The listing builds one solid part. Answer for the finished solid, in the listing's coordinates (mm). A direction names the side the tool comes from. Give positions to 0.01 mm unless a question says otherwise; leave off trailing zeros. Write each loop counter-clockwise with the first axis right and the second up, starting at its lowest first coordinate (ties: lowest second). Pieces come first, ordered by that corner, then holes. Notation, with made-up numbers: (-3, 38.25) -> (39, 38.25) arc R16 cw to (39, 50.25) -> close; hole circle Ø5 at (62.25, 64). An arc over 180 degrees is marked (long way). Write each question's results on one line, items separated by ' | '. Start each with the question number.
from build123d import *

# Parameters (mm, degrees)
F0_R      = 3.15
F1_DEPTH  = 13
F3_DEPTH  = 5.25
F5_DEPTH  = 5.5
F6_R      = 5.05
F7_DEPTH  = 5.5
F13_ANGLE = 45
F14_DEPTH = 15.67431457


# Not quite as in the source:
# - ends of sketch curves that miss each other by under 0.0002 mm in the source are joined


with BuildPart() as f1:
    # F0 (on Right) → F1 (new body, symmetric)
    with BuildSketch(Plane.YZ):
        with BuildLine():
            ThreePointArc((0.206929, -7.128644), (-5.293071, -1.628644), (0.206929, 3.871356))
            Line((0.206929, 3.871356), (17.0618508568, 3.871356))
            ThreePointArc((17.0618508568, 3.871356), (18.7952856408, 4.1814515394), (20.3137082671, 5.0732744602))
            Line((20.3137082671, 5.0732744602), (32.8624566897, 15.8173146076))
            ThreePointArc((32.8624566897, 15.8173146076), (34.1525860171, 17.5248563908), (34.6105992794, 19.6153961475))
            Line((34.6105992794, 19.6153961475), (34.6105992794, 22.815095))
            Line((34.6105992794, 22.815095), (30.788173, 22.815095))
            ThreePointArc((30.788173, 22.815095), (25.288173, 28.315095), (30.788173, 33.815095))
            Line((30.788173, 33.815095), (18.7829781294, 33.815095))
            ThreePointArc((18.7829781294, 33.815095), (17.4423484261, 33.6320143473), (16.1998960673, 33.0961797995))
            Line((16.1998960673, 33.0961797995), (-17.01485, 13.055368))
            ThreePointArc((-17.01485, 13.055368), (-20.6995911511, -1.839295663), (-32.9318010984, -11.1021976908))
            ThreePointArc((-32.9318010984, -11.1021976908), (-39.5666476125, -27.8428278397), (-21.8415422013, -31.0193857649))
            Line((-21.8415422013, -31.0193857649), (6.062198, -7.128644))
            Line((6.062198, -7.128644), (0.206929, -7.128644))
        make_face()
        with Locations((-29.405486, -22.184905)):
            Circle(F0_R, mode=Mode.SUBTRACT)
    extrude(amount=F1_DEPTH, both=True)

    # F2 (on Right) → F3 (cut, symmetric)
    with BuildSketch(Plane.YZ):
        with BuildLine():
            ThreePointArc((-21.905486, -3.502726), (-26.8533127567, -8.1227182817), (-32.9318011292, -11.1021976663))
            ThreePointArc((-32.9318011292, -11.1021976663), (-39.5869945241, -27.806130876), (-21.905486, -31.0737348541))
            Line((-21.905486, -31.0737348541), (-21.905486, -3.502726))
        make_face()
    extrude(amount=F3_DEPTH, both=True, mode=Mode.SUBTRACT)

    # F4 (on face) → F5 (cut)
    with BuildSketch(Plane.YZ.offset(13)):
        Polygon((-26.8555401867, -27.4290550439), (-23.5889459341, -22.5986621693), (-26.1388917474, -17.3545121255), (-31.9554318133, -16.9407549561), (-35.2220260659, -21.7711478307), (-32.6720802526, -27.0152978745), align=None)
    extrude(amount=-F5_DEPTH, mode=Mode.SUBTRACT)

    # F6 (on face) → F7 (cut)
    with BuildSketch(Plane(origin=(-13, 0, 0), x_dir=(0, -1, 0), z_dir=(-1, 0, 0))):
        with Locations((29.405486, -22.184905)):
            Circle(F6_R)
    extrude(amount=-F7_DEPTH, mode=Mode.SUBTRACT)

    # F8 (on Right) → F9 (revolve, cut)
    with BuildSketch(Plane.YZ):
        Polygon((30.9979878552, 13.8976717895), (-8.6011026711, 13.8976717895), (-8.6011026711, 10.921356), (-11.6011026711, 10.921356), (-11.6011026711, 12.6871454737), (-20.2870493605, 12.6871454737), (-20.375526354, 8.371356), (30.9979878552, 8.371356), align=None)
    revolve(axis=Axis((0, 5.3112307506, 8.371356), (0, -1, 0)), mode=Mode.SUBTRACT)

    # F11 (on 3pt) → F12 (revolve, cut)
    with BuildSketch(Plane(origin=(0, -33.1120649043, -10.535657015), x_dir=(-1, 0, 0), z_dir=(0, 0.95292578, 0.3032036573))):
        with BuildLine():
            Line((13, 0), (-13, 0))
            ThreePointArc((-13, 0), (0, -3.5066758251), (13, 0))
        make_face()
    revolve(axis=Axis((6.7580873147, -39.8867132027, 10.75609478), (1, 0, 0)), mode=Mode.SUBTRACT)

    # F11 (on 3pt) → F13 (revolve, cut)
    with BuildSketch(Plane(origin=(0, -33.1120649043, -10.535657015), x_dir=(-1, 0, 0), z_dir=(0, 0.95292578, 0.3032036573))):
        with BuildLine():
            Line((13, 0), (-13, 0))
            ThreePointArc((-13, 0), (0, -3.5066758251), (13, 0))
        make_face()
    revolve(axis=Axis((6.5, -29.405486, -22.184905), (1, 0, 0)), revolution_arc=F13_ANGLE, mode=Mode.SUBTRACT)

    # F14 (cut, through all): faces of the model
    f14_faces = [f1.faces().sort_by_distance(p)[0] for p in [
        (-7.6184233171, -38.9779934398, -17.2336080484),
        (7.6184233311, -38.9779934508, -17.2336080427),
    ]]
    extrude(f14_faces, amount=-F14_DEPTH, mode=Mode.SUBTRACT)


solid = f1.part
1. Section D-D (z = 29) is taken. Write down the section's boundary in (x, y), then the cut area to 3 significant figures.
2. Section C-C (x = 8.75) is taken. Write down the section's boundary in (y, z), then the cut area to 3 significant figures.
3. Section A-A (x = 0) is taken. Write down the section's boundary in (y, z).
4. A tool of negligible diameter and unlimited length cuts with its end or side. For faces 4 (the flat face through (10.29, -29.8, -27.22)), 5 (the flat face through (5.25, -34, -23)), 6 (the flat face through (-0.1, -11.601, 5.6)), 7 (the flat face through (-7.5, -32, -20)), from which of +Z, -Z, +X, -X, +Y, -Y can it reach the whole face along a straight path? Write none if from no direction.
5. Each of these flat-tipped pins is pushed along its axis until it touches: pin 1 Ø1.1 at (x, y) = (3.5, 32) entering from +Z; pin 2 Ø3 at (x, y) = (-10.5, 11) entering from -Z; pin 3 Ø8 at (x, y) = (6, 6) entering from -Z. Where does it stop, or does it pass through?
6. Section B-B (y = -18) is taken. Write down the section's boundary in (x, z), then the cut area to 3 significant figures.
7. The mould has two halves that part along Z. Classify faces 1 (the cylindrical face through (-10.29, -25.4, -25.26)), 2 (the flat face through (13, -12, 0)), 3 (the flat face through (0, 33, 22.815)): pulls with the +Z half, pulls with the -Z half, needs draft (parallel to the pull), parting line crosses it, or undercut.
8. Consider probe 1 along Y at (x, z) = (-3.75, 7); probe 2 along Z at (x, y) = (-9.5, 27); probe 3 along Z at (x, y) = (4.5, 3). Determine where each line is inside the solid, lowest interval first. Write a range as [from, to].
Results:
1) outline: (-13, 9.41) -> (13, 9.41) -> (13, 25.33) -> (-13, 25.33) -> close | area: 414 mm²
2) outline: (-41.03, -22.37) arc R11.63 ccw to (-21.84, -31.02) -> (6.06, -7.13) -> (0.21, -7.13) arc R5.5 cw to (0.21, 3.87) -> (17.06, 3.87) arc R5 ccw to (20.31, 5.07) -> (32.86, 15.82) arc R5 ccw to (34.61, 19.62) -> (34.61, 22.82) -> (30.79, 22.82) arc R5.5 cw to (30.79, 33.82) -> (18.78, 33.82) arc R5 ccw to (16.2, 33.1) -> (-15.76, 13.82) arc R24.32 cw to (-32.51, -12.42) arc R10.24 ccw to (-38.5, -17.48) -> close; hole (-35.22, -21.77) -> (-32.67, -27.02) -> (-26.86, -27.43) -> (-23.59, -22.6) -> (-26.14, -17.35) -> (-31.96, -16.94) -> close | area: 1,770 mm²
3) outline: (-21.91, -31.07) arc R11.63 ccw to (-21.84, -31.02) -> (6.06, -7.13) -> (0.21, -7.13) arc R5.5 cw to (-2.99, 2.85) -> (-8.6, 2.85) -> (-8.6, 5.82) -> (-11.6, 5.82) -> (-11.6, 4.06) -> (-14.92, 4.06) arc R25.85 cw to (-21.91, -7.82) -> close; (-14.33, 14.67) arc R25.85 cw to (-14.11, 12.69) -> (-11.6, 12.69) -> (-11.6, 10.92) -> (-8.6, 10.92) -> (-8.6, 13.9) -> (30.62, 13.9) -> (32.86, 15.82) arc R5 ccw to (34.61, 19.62) -> (34.61, 22.82) -> (30.79, 22.82) arc R5.5 cw to (30.79, 33.82) -> (18.78, 33.82) arc R5 ccw to (16.2, 33.1) -> close
4) face 4: +X | face 5: +Z, -Z, -Y | face 6: -Y | face 7: -X
5) pin 1: stops at z = 22.82 | pin 2: stops at z = 3.87 | pin 3: stops at z = -10.61
6) outline: (-13, -27.73) -> (13, -27.73) -> (13, 3.8) -> (11.87, 3.8) arc R13.76 cw to (-11.87, 3.8) -> (-13, 3.8) -> close | area: 705 mm²
7) face 1: undercut | face 2: needs draft | face 3: pulls with the +Z half
8) probe 1: y = [-11.6, -8.6] | probe 2: z = [10.8, 24.33], [32.3, 33.82] | probe 3: z = [-9.75, -7.13], [3.87, 5.16], [11.58, 25.13]
